Can you work these out from the drawing? Everything is in mm from the part's minimum corner. A direction names the side the tool comes from. Round coordinates to 2 decimals unless told otherwise and drop trailing zeros. Loops run counter-clockwise (first coordinate to the right, second up) from the corner with the lowest first, then second, coordinate; pieces in that order, holes last. Notation, with made-up numbers: M -27.75,70 L -3.75,70 A19 cw -3.75,102 Z; hole C 49,67 d5. An arc over 180 degrees is marked long. Use a Markdown table: item, result.
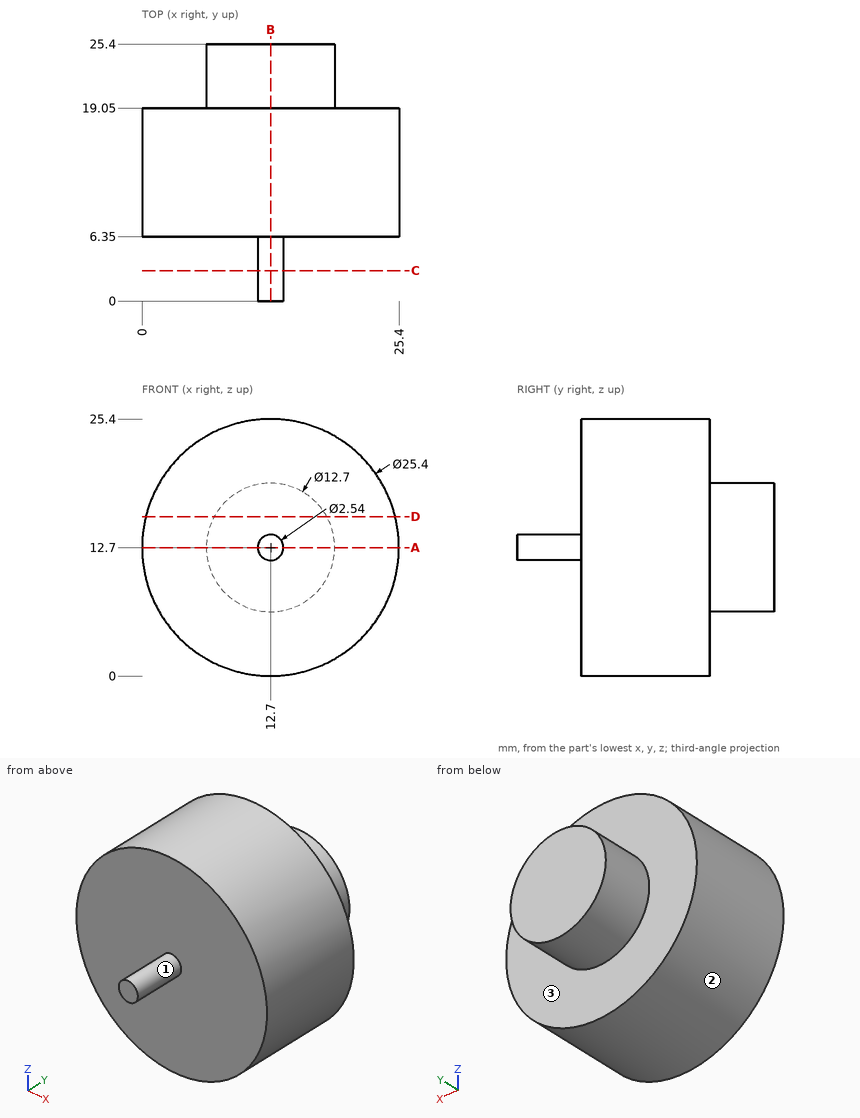
Q1. Imagine slicing it at C-C, the plane y = 3. Please give me the cut outline in (x, z), then the cut area to 3 significant figures.
Return value:
| item | result |
|---|---|
| outline | C 12.7,12.7 d2.54 |
| area | 5.07 mm^2 |
Q2. For the marked faces 1, 2 and 3, which set-ups out of +Z, -Z, +X, -X, +Y, -Y let a thin tool reach every point of the face, with its end or its side?
Return value:
| item | result |
|---|---|
| face 1 | -Y |
| face 2 | +Y, -Y |
| face 3 | +Y |
Q3. Imagine slicing it at B-B, the plane x = 12.7. Please give me the cut outline in (y, z), then the cut area to 3 significant figures.
Return value:
| item | result |
|---|---|
| outline | M 0,11.43 L 6.35,11.43 L 6.35,0 L 19.05,0 L 19.05,6.35 L 25.4,6.35 L 25.4,19.05 L 19.05,19.05 L 19.05,25.4 L 6.35,25.4 L 6.35,13.97 L 0,13.97 Z |
| area | 419 mm^2 |
Q4. Imagine slicing it at D-D, the plane z = 15.75. Please give me the cut outline in (x, y).
Return value:
| item | result |
|---|---|
| outline | M 0.37,6.35 L 25.03,6.35 L 25.03,19.05 L 18.27,19.05 L 18.27,25.4 L 7.13,25.4 L 7.13,19.05 L 0.37,19.05 Z |
Q5. Imagine slicing it at A-A, the plane z = 12.7. Please give me the cut outline in (x, y), then the cut area to 3 significant figures.
Return value:
| item | result |
|---|---|
| outline | M 0,6.35 L 11.43,6.35 L 11.43,0 L 13.97,0 L 13.97,6.35 L 25.4,6.35 L 25.4,19.05 L 19.05,19.05 L 19.05,25.4 L 6.35,25.4 L 6.35,19.05 L 0,19.05 Z |
| area | 419 mm^2 |
Q6. Will these pins go through, and if not, where does the flat tip stop? P1, Ø5, axis at y = 7, z = 20, coming from the +X side; P2, Ø12, axis at y = 8, z = 10.5, coming from the +X side; P3, Ø8, axis at y = 12, z = 18, coming from the +X side; P4, Ø5, axis at y = 6.5, z = 21.5, coming from the +X side.
Return value:
| item | result |
|---|---|
| P1 | stops at x = 24.46 |
| P2 | stops at x = 25.4 |
| P3 | stops at x = 25.33 |
| P4 | stops at x = 23.73 |
Q7. I need wall thicknesses on line 1 (Y direction, x = 11.5, z = 16); line 2 (Y direction, x = 11.5, z = 3.75); line 3 (X direction, y = 13.25, z = 21). Which ranges of each line are inside material? Lowest first, please. Write a range as from..to.
Return value:
| item | result |
|---|---|
| line 1 | y = 6.35..25.4 |
| line 2 | y = 6.35..19.05 |
| line 3 | x = 3.09..22.31 |
